Could you check a few things on this model? Use its own coordinates, in mm. A direction names the side the tool comes from. Round coordinates to 2 decimals unless told otherwise and drop trailing zeros. Write each loop counter-clockwise with the first axis right and the second up, starting at its lowest first coordinate (ties: lowest second). Pieces come first, ordered by that corner, then holes. Notation, with made-up numbers: (70.5, 55) -> (107.5, 55) arc R5 ccw to (107.5, 62) -> close; hole circle Ø11 at (51, 78). An arc over 180 degrees is marked (long way). Return JSON: item names as keys, results as strings.
from build123d import *


with BuildPart() as f1:
    # F0 (on Top) → F1 (revolve)
    with BuildSketch(Plane.XY):
        with BuildLine():
            Line((131.669218, 0), (-91.342782, 0))
            Line((-91.342782, 0), (-91.342782, -99.949))
            Line((-91.342782, -99.949), (-65.942782, -99.949))
            ThreePointArc((-65.942782, -99.949), (-55.483238, -103.202239), (-48.714109, -111.814122))
            Line((-48.714109, -111.814122), (-32.371455, -154.631878))
            ThreePointArc((-32.371455, -154.631878), (-25.602327, -163.243761), (-15.142782, -166.497))
            Line((-15.142782, -166.497), (55.469218, -166.497))
            ThreePointArc((55.469218, -166.497), (65.928762, -163.243761), (72.697891, -154.631878))
            Line((72.697891, -154.631878), (89.040545, -111.814122))
            ThreePointArc((89.040545, -111.814122), (95.809673, -103.202239), (106.269218, -99.949))
            Line((106.269218, -99.949), (131.669218, -99.949))
            Line((131.669218, -99.949), (131.669218, 0))
        make_face()
    revolve(axis=Axis((20.163218, 0, 0), (1, 0, 0)))


solid = f1.part
1) I want a section at D-D, the plane x = -43.5. Please give me the cut outline in (y, z), and give its area (3 significant figures).
Return value:
{"outline": "circle Ø250.95 at (0, 0)", "area": "49,500 mm²"}
2) I want a section at A-A, the plane z = 0. Please give me the cut outline in (x, y).
Return value:
{"outline": "(-91.34, -99.95) -> (-65.94, -99.95) arc R18.44 cw to (-48.71, -111.81) -> (-32.37, -154.63) arc R18.44 ccw to (-15.14, -166.5) -> (55.47, -166.5) arc R18.44 ccw to (72.7, -154.63) -> (89.04, -111.81) arc R18.44 cw to (106.27, -99.95) -> (131.67, -99.95) -> (131.67, 99.95) -> (106.27, 99.95) arc R18.44 cw to (89.04, 111.81) -> (72.7, 154.63) arc R18.44 ccw to (55.47, 166.5) -> (-15.14, 166.5) arc R18.44 ccw to (-32.37, 154.63) -> (-48.71, 111.81) arc R18.44 cw to (-65.94, 99.95) -> (-91.34, 99.95) -> close"}
3) Thinking about a two-plate mould opening in Y: for faces 4 (the face through (88.25, 14.83, -112.92)), 5 (the face through (-91.343, -1, -1)), which applies, pulls with the +Y half, pulls with the -Y half, needs draft (parallel to the pull), parting line crosses it, or undercut?
Return value:
{"face 4": "parting line crosses it", "face 5": "needs draft"}
4) Will these pins go through, and if not, where does the flat tip stop? pin 1 Ø3 at (x, y) = (-12, -45) entering from -Z; pin 2 Ø6 at (x, z) = (-13, 115) entering from +Y; pin 3 Ø12 at (x, y) = (9, -94) entering from -Z.
Return value:
{"pin 1": "z = -160.71", "pin 2": "y = 123.2", "pin 3": "z = -141.34"}
5) If I drill on probe 1 along Z at (x, y) = (62.5, 116); probe 2 along Y at (x, z) = (98.5, 21); probe 3 along Y at (x, z) = (9.5, -126), over which ranges is the centre line in solid material (lowest first)? Write a range as [from, to].
Return value:
{"probe 1": "[-117.49, 117.49]", "probe 2": "[-99.47, 99.47]", "probe 3": "[-108.84, 108.84]"}
6) For faces 1 (the face through (119.147, -95.334, -30.022)), 2 (the face through (-78.465, -95.334, -30.022)), 3 (the face through (20.66, 21.67, -165.08)), which set-ups out of +Z, -Z, +X, -X, +Y, -Y let a thin tool reach every point of the face, with its end or its side?
Return value:
{"face 1": "+X", "face 2": "-X", "face 3": "+X, -X"}
7) I want a section at C-C, the plane x = 27.5. Please give me the cut outline in (y, z).
Return value:
{"outline": "circle Ø332.99 at (0, 0)"}
